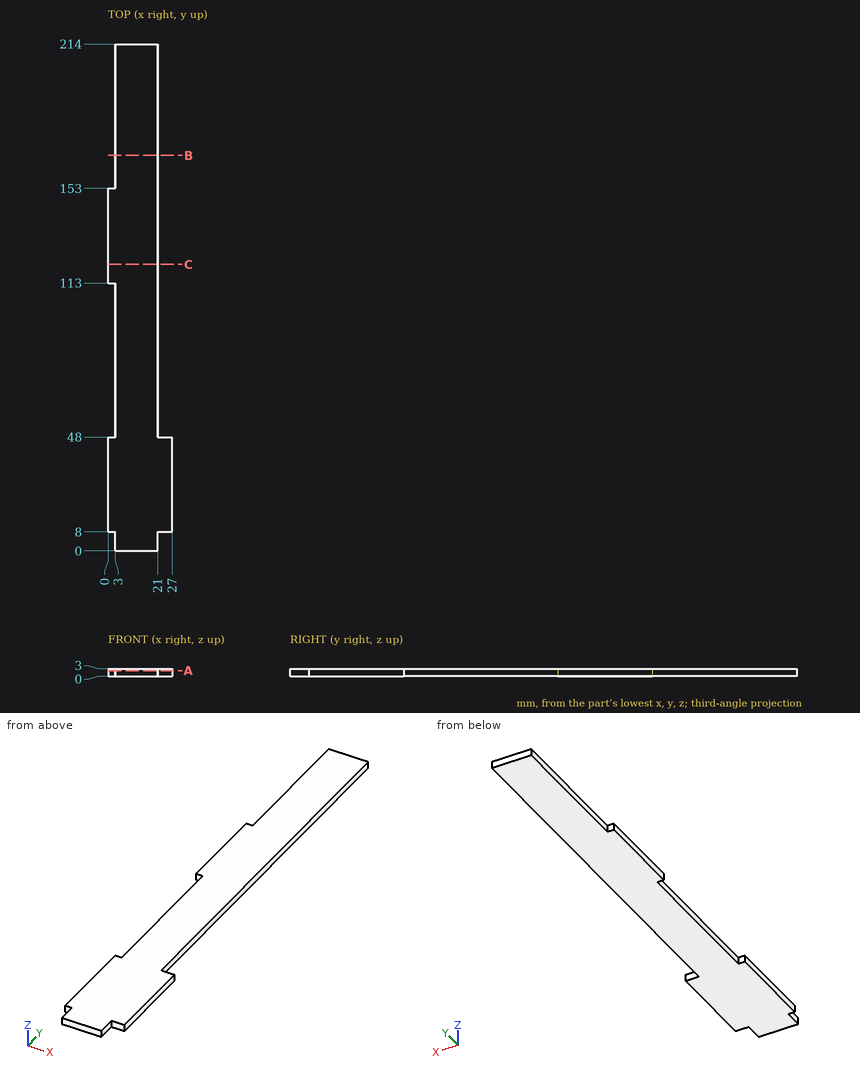
Study the drawing (mm; zero at the part's minimum x, y, z) and answer. Give positions to 0.01 mm unless a question says otherwise; leave off trailing zeros. Loops run counter-clockwise (first coordinate to the right, second up) from the corner with the lowest first, then second, coordinate; pieces in that order, holes last. Notation, with made-up numbers: M -38.5,-4 L -15.5,-4 A34 ccw -15.5,33 Z; hole C 21.5,-30.5 d4. An arc over 180 degrees is marked long. Use CSV: the item, a comma, the result in double quotes.
1) Find section B-B on y = 167. Write down the section's boundary in (x, z), plus the area to 3 significant figures.
Answer:
outline,"M 3,0 L 21,0 L 21,3 L 3,3 Z"
area,"54.0 mm^2"
2) Find section A-A on z = 2.3. Write down the section's boundary in (x, y), plus the area to 3 significant figures.
Answer:
outline,"M 0,8 L 3,8 L 3,0 L 21,0 L 21,8 L 27,8 L 27,48 L 21,48 L 21,214 L 3,214 L 3,153 L 0,153 L 0,113 L 3,113 L 3,48 L 0,48 Z"
area,"4,330 mm^2"
3) Find section C-C on y = 121. Write down the section's boundary in (x, z).
Answer:
outline,"M 0,0 L 21,0 L 21,3 L 0,3 Z"
4) Given P1, Ø1.5, axis at y = 100, z = 1.5, coming from the +X side; P2, Ø3, axis at x = 2.5, y = 106.5, coming from the +Z side; P3, Ø0.9, axis at x = 25, z = 1.5, coming from the -Y side; P4, Ø0.9, axis at x = 24, z = 1.5, coming from the +Y side, each flat-ended and moving along its own axis, determine where each tip first touches the part or whether it passes through.
Answer:
P1,"x = 21"
P2,"z = 3"
P3,"y = 8"
P4,"y = 48"
5) Consider L1, parallel to X at y = 132.5, z = 0.6; L2, parallel to Y at x = 1.75, z = 2; L3, parallel to Y at x = 23.5, z = 2.5. Determine where each line is inside the solid, lowest interval first.
Answer:
L1,"0 to 21"
L2,"8 to 48, 113 to 153"
L3,"8 to 48"
